Geometry check sheet. Reference: the model listing, model coordinates, mm. A direction names the side the tool comes from. Coordinates: 2 decimals unless noted, no trailing zeros. Write each loop counter-clockwise with the first axis right and the second up, starting at its lowest first coordinate (ties: lowest second). Pieces come first, ordered by that corner, then holes. Notation, with made-up numbers: (0, 89.5) -> (45, 89.5) arc R14 ccw to (45, 113.5) -> close; hole circle Ø10 at (63.25, 55.25). An arc over 180 degrees is marked (long way). Put each result on its own line as item: value. Start each with the question number.
from build123d import *

# Parameters (mm, degrees)
SKETCH_1_R      = 1.5
EXTRUDE_1_DEPTH = 14
SKETCH_2_R      = 1.5
EXTRUDE_2_DEPTH = 7


with BuildPart() as part:
    # 草图1 → 凸台-拉伸1 (new body)
    with BuildSketch(Plane(origin=(0, 0, 0), x_dir=(0, 0, -1), z_dir=(1, 0, 0))):
        Circle(SKETCH_1_R)
    extrude(amount=EXTRUDE_1_DEPTH)

    # 草图2 → 凸台-拉伸2 (add, symmetric)
    with BuildSketch(Plane.XY):
        with Locations(Location((7, 0, 0), (0, 0, 90))):
            Circle(SKETCH_2_R)
    extrude(amount=EXTRUDE_2_DEPTH, both=True)


solid = part.part
Item 1: Section check B-B, the plane z = -1. Enter the section's corners in (x, y), and give its area (3 significant figures).
Item 2: Section check D-D, the plane z = 2. Enter the section's corners in (x, y).
Item 3: Access from +Z, -Z, +X, -X, +Y, -Y to the whole of each face (thin tool, end or side, straight path). Record for faces 1 (the cylindrical face through (2.67, 0.07, 1.5)), 2 (the cylindrical face through (11.23, 1.01, 1.11)), 3 (the cylindrical face through (6.93, -1.5, -4.23)), 4 (the cylindrical face through (6.93, -1.5, 4.33)).
Item 4: Section check C-C, the plane x = 9.5. Enter the section's corners in (y, z), and give its area (3 significant figures).
Item 5: Scan lines: line 1 along X through (y, z) = (0.05, 2.75); line 2 along Z through (x, y) = (3.25, -0.1); line 3 along X through (y, z) = (0.65, -3). Record each from-to range of solid material in increasing order. Write a range as [from, to].
Item 6: Go/stop test with flat-tipped pins: P1, Ø1, axis at x = 10, z = -2.5, coming from the -Y side; P2, Ø1.5, axis at x = 12.5, y = 0, coming from the +Z side; P3, Ø1, axis at y = -0.5, z = 4, coming from the +X side; P4, Ø4, axis at x = 12.5, z = 3, coming from the -Y side. Record where each tip stops, or that it passes through.
Item 7: Section check A-A, the plane y = 0. Enter the section's corners in (x, z).
From the geometry:
1. outline: (0, -1.12) -> (6, -1.12) arc R1.5 ccw to (8, -1.12) -> (14, -1.12) -> (14, 1.12) -> (8, 1.12) arc R1.5 ccw to (6, 1.12) -> (0, 1.12) -> close
1. area: 32.4 mm²
2. outline: circle Ø3 at (7, 0)
3. face 1: -X
3. face 2: +X
3. face 3: -Z
3. face 4: +Z
4. outline: circle Ø3 at (0, 0)
4. area: 7.07 mm²
5. line 1: [5.5, 8.5]
5. line 2: [-1.5, 1.5]
5. line 3: [5.65, 8.35]
6. P1: through
6. P2: z = 1.5
6. P3: x = 8.5
6. P4: y = -1.12
7. outline: (0, -1.5) -> (5.5, -1.5) -> (5.5, -7) -> (8.5, -7) -> (8.5, -1.5) -> (14, -1.5) -> (14, 1.5) -> (8.5, 1.5) -> (8.5, 7) -> (5.5, 7) -> (5.5, 1.5) -> (0, 1.5) -> close
